from build123d import *

# Parameters (mm, degrees)
SKETCH1_R               = 4
BOSS_EXTRUDE1_DEPTH     = 5
BOSS_EXTRUDE2_START     = 1
BOSS_EXTRUDE2_DEPTH     = 1
SKETCH3_R               = 0.4
CUT_EXTRUDE1_DEPTH      = 1
CUT_EXTRUDE1_DEPTH_BACK = 6


with BuildPart() as part:
    # Sketch1 → Boss-Extrude1 (new body)
    with BuildSketch(Plane(origin=(0, 0, 0), x_dir=(1, 0, 0), z_dir=(0, 1, 0))):
        Circle(SKETCH1_R)
    extrude(amount=BOSS_EXTRUDE1_DEPTH)

    # Sketch2 → Boss-Extrude2 (add)
    with BuildSketch(Plane(origin=(0, 0, 0), x_dir=(1, 0, 0), z_dir=(0, 1, 0)).offset(BOSS_EXTRUDE2_START)):
        with BuildLine():
            Line((15, -2), (3.464101615, -2))
            ThreePointArc((3.464101615, -2), (4, 0), (3.464101615, 2))
            add(Edge.make_bspline(
                [(3.464101615, 2), (7.059911859, 2.261875705), (11.549393059, 4.995376959), (15, 2)],
                knots=[0, 0, 0, 0, 1, 1, 1, 1], degree=3))
            Line((15, 2), (15, 0))
            Line((15, 0), (15, -2))
        make_face()
        with BuildLine():
            Line((2, -15), (0, -15))
            Line((0, -15), (-2, -15))
            Line((-2, -15), (-2, -3.464101615))
            ThreePointArc((-2, -3.464101615), (0, -4), (2, -3.464101615))
            add(Edge.make_bspline(
                [(2, -3.464101615), (2.261875705, -7.059911859), (4.995376959, -11.549393059), (2, -15)],
                knots=[0, 0, 0, 0, 1, 1, 1, 1], degree=3))
        make_face()
        with BuildLine():
            Line((-15, -2), (-15, 0))
            Line((-15, 0), (-15, 2))
            Line((-15, 2), (-3.464101615, 2))
            ThreePointArc((-3.464101615, 2), (-4, 0), (-3.464101615, -2))
            add(Edge.make_bspline(
                [(-3.464101615, -2), (-7.059911859, -2.261875705), (-11.549393059, -4.995376959), (-15, -2)],
                knots=[0, 0, 0, 0, 1, 1, 1, 1], degree=3))
        make_face()
        with BuildLine():
            Line((-2, 15), (0, 15))
            Line((0, 15), (2, 15))
            Line((2, 15), (2, 3.464101615))
            ThreePointArc((2, 3.464101615), (0, 4), (-2, 3.464101615))
            add(Edge.make_bspline(
                [(-2, 3.464101615), (-2.261875705, 7.059911859), (-4.995376959, 11.549393059), (-2, 15)],
                knots=[0, 0, 0, 0, 1, 1, 1, 1], degree=3))
        make_face()
    extrude(amount=BOSS_EXTRUDE2_DEPTH)

    # Sketch3 → Cut-Extrude1 (cut, two sides)
    with BuildSketch(Plane(origin=(0, 5, 0), x_dir=(1, 0, 0), z_dir=(0, 1, 0))) as cut_extrude1_sk:
        Circle(SKETCH3_R)
    extrude(amount=CUT_EXTRUDE1_DEPTH, mode=Mode.SUBTRACT)
    extrude(cut_extrude1_sk.sketch, amount=-CUT_EXTRUDE1_DEPTH_BACK, mode=Mode.SUBTRACT)


solid = part.part
Design review of the part built by this model. Coordinates are the model's own, in mm. A direction names the side the tool comes from. Coordinates: 2 decimals unless noted, no trailing zeros. Loops run counter-clockwise (first coordinate to the right, second up) from the corner with the lowest first, then second, coordinate; pieces in that order, holes last.
Item 1: Add section C-C (y = 3.75). Write out the cut boundary in (x, z).
Completed:
outline: circle Ø8 at (0, 0); hole circle Ø0.8 at (0, 0)
Item 2: Clearance check with flat-ended pins moving along their axes: pin 1 (1.6 mm diameter, centred on x = -1, z = -7.5, fed in from +Y); pin 2 (1.1 mm diameter, centred on x = 11, y = 1.5, fed in from +Z); pin 3 (2.5 mm diameter, centred on x = 0.5, z = -12, fed in from -Y). State where each tip first meets the part, or that it passes through.
Completed:
pin 1: stops at y = 2
pin 2: stops at z = 2
pin 3: stops at y = 1
Item 3: Wall thickness on L1, parallel to X at y = 4, z = 0; L2, parallel to Z at x = 0, y = 1.7: over which ranges is each line inside the solid? List them lowest first.
Completed:
L1: x = -4 to -0.4, 0.4 to 4
L2: z = -15 to -0.4, 0.4 to 15
Item 4: For faces 1 (the flat face through (2, 1.5, -9.3)), 2 (the flat face through (-2, 1.5, 9.3)), 3 (the cylindrical face through (-2.95, 2.46, -2.7)), 4 (the flat face through (-9.3, 1.5, -2)), list the 3-axis set-ups (+Z, -Z, +X, -X, +Y, -Y) from which the entire face can be reached by the end or side of a thin tool; tool diameter is ignored.
Completed:
face 1: -Z, +X, +Y, -Y
face 2: +Z, -X, +Y, -Y
face 3: none
face 4: -Z, -X, +Y, -Y
Item 5: Add section B-B (x = 0). Write out the cut boundary in (y, z), and give its area (3 significant figures).
Completed:
outline: (0, -4) - (1, -4) - (1, -15) - (2, -15) - (2, -4) - (5, -4) - (5, -0.4) - (0, -0.4) - close; (0, 0.4) - (5, 0.4) - (5, 4) - (2, 4) - (2, 15) - (1, 15) - (1, 4) - (0, 4) - close
area: 58.0 mm2
Item 6: Add section A-A (z = 0). Write out the cut boundary in (x, y), and give its area (3 significant figures).
Completed:
outline: (-15, 1) - (-4, 1) - (-4, 0) - (-0.4, 0) - (-0.4, 5) - (-4, 5) - (-4, 2) - (-15, 2) - close; (0.4, 0) - (4, 0) - (4, 1) - (15, 1) - (15, 2) - (4, 2) - (4, 5) - (0.4, 5) - close
area: 58.0 mm2
